from build123d import *

# Parameters (mm, degrees)
SKETCH3_R           = 16
BOSS_EXTRUDE1_DEPTH = 80
SKETCH4_R           = 36
BOSS_EXTRUDE2_DEPTH = 38
FILLET1_R           = 3


with BuildPart() as part:
    # Sketch3 → Boss-Extrude1 (new body)
    with BuildSketch(Plane(origin=(0, 0, 0), x_dir=(0, 0, -1), z_dir=(1, 0, 0))):
        Circle(SKETCH3_R)
    extrude(amount=BOSS_EXTRUDE1_DEPTH)

    # Sketch4 → Boss-Extrude2 (add)
    with BuildSketch(Plane(origin=(80, 0, 0), x_dir=(0, 0, -1), z_dir=(1, 0, 0))):
        Circle(SKETCH4_R)
    extrude(amount=BOSS_EXTRUDE2_DEPTH)

    # Fillet1
    fillet1_edges = [part.edges().sort_by_distance(p)[0] for p in [
        (0, 0, 16),
        (80, 0, 16),
    ]]
    fillet(fillet1_edges, radius=FILLET1_R)


solid = part.part
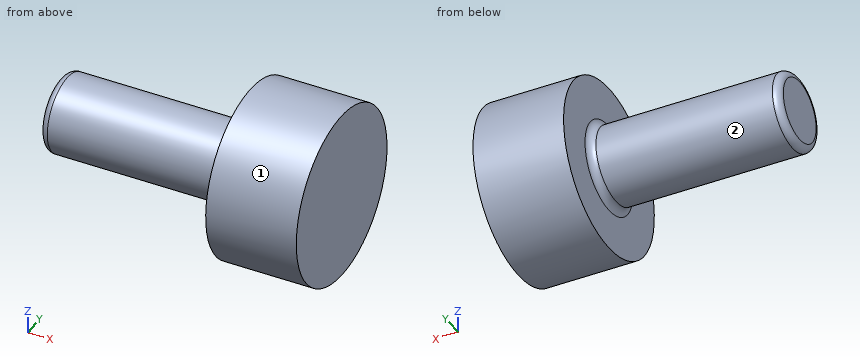
For this review, take the finished solid that the model builds, in its own axes (mm). Face numbers are marked on the shaded views. A direction names the side the tool comes from. Give positions to 0.01 mm unless a question says otherwise; leave off trailing zeros. Loops run counter-clockwise (first coordinate to the right, second up) from the corner with the lowest first, then second, coordinate; pieces in that order, holes last. Notation, with made-up numbers: M 19,54.25 L 59,54.25 A17 cw 59,65.25 Z; hole C 40.5,53.5 d10. An arc over 180 degrees is marked long. Put each result on its own line as item: value. Start each with the question number.
(1) For pin 1 (2 mm diameter, centred on y = 13, z = -15.5, fed in from -X); pin 2 (4 mm diameter, centred on x = 36, y = 9, fed in from +Z); pin 3 (2 mm diameter, centred on x = 66, y = 0, fed in from -Z), all flat-tipped, find the tip position at first contact; note any pin that passes through.
(2) Add section A-A, the plane y = 0. Write out the cut boundary in (x, z), then the cut area to 3 significant figures.
(3) Add section C-C, the plane x = 96.5. Write out the cut boundary in (y, z).
(4) Wall thickness on L1, parallel to X at y = 21, z = -8.5; L2, parallel to Y at x = 95, z = -33; L3, parallel to Y at x = 50.5, z = 3: over which ranges is each line inside the solid? List them lowest first.
(5) Machinability: for the marked faces 1 and 2, which of the approach directions +Z, -Z, +X, -X, +Y, -Y give a long, thin tool a straight path to every point of the face, cutting with its end or side? Answer none if there is none.
(6) Add section D-D, the plane x = 44.5. Write out the cut boundary in (y, z), then the cut area to 3 significant figures.
Result:
1. pin 1: stops at x = 80
1. pin 2: stops at z = 14.39
1. pin 3: stops at z = -16
2. outline: M 0,-13 A3 ccw 3,-16 L 77,-16 A3 cw 80,-19 L 80,-36 L 118,-36 L 118,36 L 80,36 L 80,19 A3 cw 77,16 L 3,16 A3 ccw 0,13 Z
2. area: 5,300 mm^2
3. outline: C 0,0 d72
4. L1: x = 80 to 118
4. L2: y = -14.39 to 14.39
4. L3: y = -15.72 to 15.72
5. face 1: +X, -X
5. face 2: -X
6. outline: C 0,0 d32
6. area: 804 mm^2
